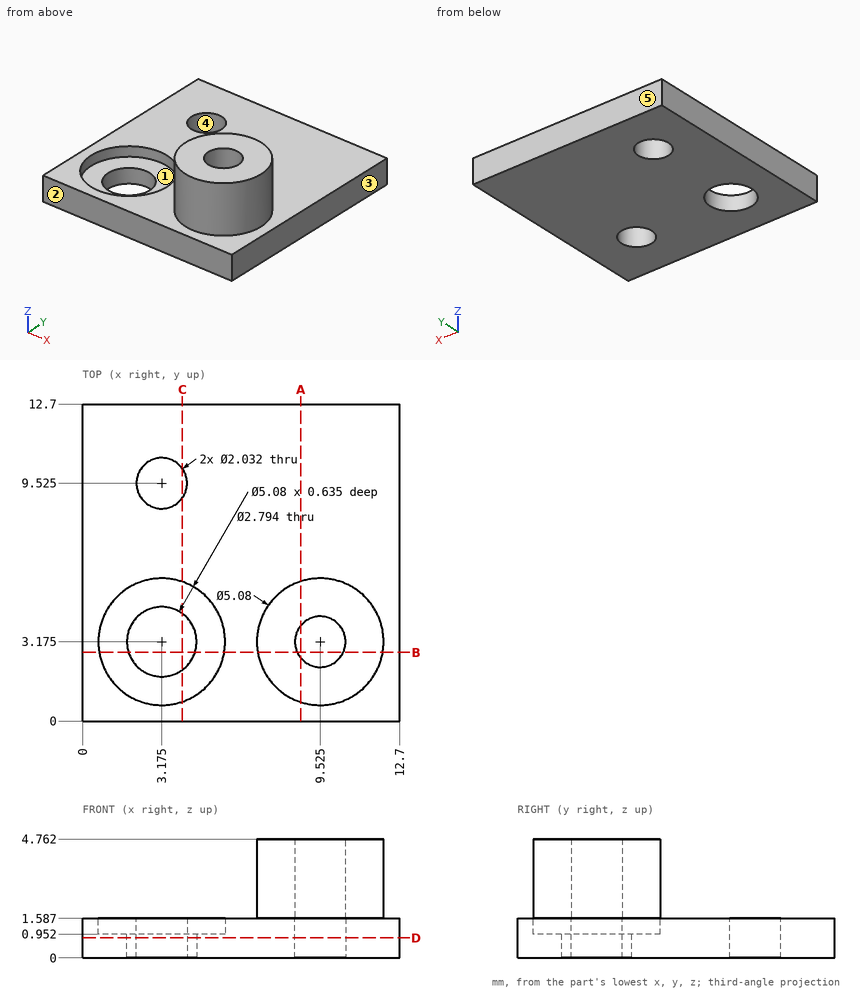
Job drawing, mm, ordinate dimensions from the low corner. One solid piece. A direction names the side the tool comes from. Round coordinates to 2 decimals unless told otherwise and drop trailing zeros. Order: outer loops, then holes, each group sorted by start corner. A loop starts at its lowest first (then second) coordinate and runs counter-clockwise, first axis right, second up. Notation, with made-up numbers: (-37.75, -19) -> (-23.75, -19) arc R23 cw to (-23.75, 19) -> close; hole circle Ø5 at (70.25, 80). An arc over 180 degrees is marked (long way). Write item = value, one per line.
(1) Pull direction Y, two halves, no side cores. Call the marked faces 3, 4 and 5: +Y half, -Y half, draft (parallel to the pull), parting line (faces both ways), or undercut.
Answers follow:
face_3 = draft
face_4 = undercut
face_5 = +Y half
(2) Cut at C-C (x = 4). Write the cut outline in (y, z).
Answers follow:
outline = (0, 0) -> (2.05, 0) -> (2.05, 0.95) -> (0.77, 0.95) -> (0.77, 1.59) -> (0, 1.59) -> close; (4.3, 0) -> (8.93, 0) -> (8.93, 1.59) -> (5.58, 1.59) -> (5.58, 0.95) -> (4.3, 0.95) -> close; (10.12, 0) -> (12.7, 0) -> (12.7, 1.59) -> (10.12, 1.59) -> close
(3) 3-axis set-ups, long thin cutter, end or side, ignore diameter. For the marked faces 1 and 2: which of +Z, -Z, +X, -X, +Y, -Y reach the whole face in a straight line?
Answers follow:
face_1 = +Z
face_2 = +Z, -Z, +X, -X, -Y
(4) Cut at B-B (y = 2.75). Write the cut outline in (x, z) (1 decimal).
Answers follow:
outline = (0, 0) -> (1.8, 0) -> (1.8, 1) -> (0.7, 1) -> (0.7, 1.6) -> (0, 1.6) -> close; (4.5, 0) -> (8.6, 0) -> (8.6, 4.8) -> (7, 4.8) -> (7, 1.6) -> (5.7, 1.6) -> (5.7, 1) -> (4.5, 1) -> close; (10.4, 0) -> (12.7, 0) -> (12.7, 1.6) -> (12, 1.6) -> (12, 4.8) -> (10.4, 4.8) -> close
(5) Drill centre lines: L1, parallel to Y at x = 3, z = 1.2 (1 decimal); L2, parallel to Y at x = 9.5, z = 0.85; L3, parallel to X at y = 3.5, z = 0.8 (1 decimal). Where is each one in solid material? Low to high.
Answers follow:
L1 = 0 to 0.6, 5.7 to 8.5, 10.5 to 12.7
L2 = 0 to 2.16, 4.19 to 12.7
L3 = 0 to 1.8, 4.5 to 8.6, 10.5 to 12.7
(6) Flat gauge pins, fed straight in: P1, Ø4, axis at x = 2, y = 2.5, coming from the +Z side; P2, Ø3, axis at x = 3.175, y = 3.175, coming from the +Z side. Where does each tip first touch, or does it go through?
Answers follow:
P1 = 1.59
P2 = 0.95
(7) Cut at A-A (x = 8.75). Write the cut outline in (y, z).
Answers follow:
outline = (0, 0) -> (2.52, 0) -> (2.52, 4.76) -> (0.76, 4.76) -> (0.76, 1.59) -> (0, 1.59) -> close; (3.83, 0) -> (12.7, 0) -> (12.7, 1.59) -> (5.59, 1.59) -> (5.59, 4.76) -> (3.83, 4.76) -> close
(8) Cut at D-D (z = 0.8). Write the cut outline in (x, y) (1 decimal), plus the area to 3 significant figures.
Answers follow:
outline = (0, 0) -> (12.7, 0) -> (12.7, 12.7) -> (0, 12.7) -> close; hole circle Ø2.8 at (3.2, 3.2); hole circle Ø2 at (3.2, 9.5); hole circle Ø2 at (9.5, 3.2)
area = 149 mm²
